Geometry check sheet. Reference: the model listing, model coordinates, mm. A direction names the side the tool comes from. Round coordinates to 2 decimals unless told otherwise and drop trailing zeros. Loops run counter-clockwise (first coordinate to the right, second up) from the corner with the lowest first, then second, coordinate; pieces in that order, holes last. Notation, with made-up numbers: (-22.5, -24.5) - (34.5, -24.5) arc R10 ccw to (34.5, -8.5) - close; hole circle Ø2 at (33.5, 18.5). An arc over 180 degrees is marked (long way). Write item = value, one per line.
```python
from build123d import *

# Parameters (mm, degrees)
SKETCH1_R           = 35
SKETCH1_R_2         = 11.65
BOSS_EXTRUDE1_DEPTH = 4
CUT_EXTRUDE1_DEPTH  = 10
SKETCH6_R           = 1
CUT_EXTRUDE4_DEPTH  = 10
BOSS_EXTRUDE3_START = 1
SKETCH7_R           = 11.65
SKETCH7_R_2         = 10.65
BOSS_EXTRUDE3_DEPTH = 1
SKETCH8_R           = 11.65
SKETCH8_R_2         = 11.15
CUT_EXTRUDE5_DEPTH  = 0.25
FILLET1_R           = 0.1
CUT_EXTRUDE6_DEPTH  = 1


with BuildPart() as part:
    # Sketch1 → Boss-Extrude1 (new body)
    with BuildSketch(Plane(origin=(0, 0, 0), x_dir=(0, -0.16775650988153862, -0.9858284604292805), z_dir=(1, 0, 0))):
        with Locations(Location((-28.542888787, 18.957113921, 0), (0, 0, 9.65740334))):
            Circle(SKETCH1_R)
        with Locations(Location((-28.542888787, 18.957113921, 0), (0, 0, 9.65740334))):
            Circle(SKETCH1_R_2, mode=Mode.SUBTRACT)
    extrude(amount=BOSS_EXTRUDE1_DEPTH)

    # Sketch2 → Cut-Extrude1 (cut)
    with BuildSketch(Plane.ZY):
        with BuildLine():
            Line((38.375552951, 38.308271509), (48.999843401, 48.932561958))
            Line((48.999843401, 48.932561958), (51.312030188, 52.930544456))
            Line((51.312030188, 52.930544456), (54.007279042, 51.111570475))
            Line((54.007279042, 51.111570475), (50.414056963, 47.518348396))
            Line((50.414056963, 47.518348396), (39.789766514, 36.894057946))
            ThreePointArc((39.789766514, 36.894057946), (39.100348464, 37.618853459), (38.375552951, 38.308271509))
        make_face()
    extrude(amount=-CUT_EXTRUDE1_DEPTH, mode=Mode.SUBTRACT)

    # Sketch6 → Cut-Extrude4 (cut)
    with BuildSketch(Plane(origin=(4, 0, 0), x_dir=(0, 0, -1), z_dir=(1, 0, 0))):
        with Locations((-24.958212841, -4.023282164)):
            Circle(SKETCH6_R)
        with Locations((2.541787159, 23.476717836)):
            Circle(SKETCH6_R)
        with Locations((-52.458212841, 23.476717836)):
            Circle(SKETCH6_R)
        with Locations((-24.958212841, 50.976717836)):
            Circle(SKETCH6_R)
    extrude(amount=-CUT_EXTRUDE4_DEPTH, mode=Mode.SUBTRACT)

    # Sketch7 → Boss-Extrude3 (add)
    with BuildSketch(Plane.ZY.offset(-4).offset(BOSS_EXTRUDE3_START)):
        with Locations((24.958212841, 23.476717836)):
            Circle(SKETCH7_R)
        with Locations((24.958212841, 23.476717836)):
            Circle(SKETCH7_R_2, mode=Mode.SUBTRACT)
    extrude(amount=-BOSS_EXTRUDE3_DEPTH)

    # Sketch8 → Cut-Extrude5 (cut)
    with BuildSketch(Plane.ZY.offset(-3)):
        with Locations((24.958212841, 23.476717836)):
            Circle(SKETCH8_R)
        with Locations((24.958212841, 23.476717836)):
            Circle(SKETCH8_R_2, mode=Mode.SUBTRACT)
    extrude(amount=-CUT_EXTRUDE5_DEPTH, mode=Mode.SUBTRACT)

    # Fillet1
    fillet1_edges = [part.edges().sort_by_distance(p)[0] for p in [
        (3.25, 23.476717836, 13.808212841),
    ]]
    fillet(fillet1_edges, radius=FILLET1_R)

    # Sketch9 → Cut-Extrude6 (cut)
    with BuildSketch(Plane.ZY):
        Polygon((36.254232608, 38.308271509), (48.989739813, 51.043778714), (52.525273719, 47.508244808), (39.789766514, 34.772737603), (39.082659732, 34.065630822), (35.547125827, 37.601164728), align=None)
        Polygon((48.989739813, 48.922458371), (50.403953376, 47.508244808), (40.402946038, 37.507237471), (38.988732476, 38.921451033), align=None, mode=Mode.SUBTRACT)
    extrude(amount=-CUT_EXTRUDE6_DEPTH, mode=Mode.SUBTRACT)


solid = part.part
```
(1) Section check C-C (z = 9.5). Enter the section's corners in (x, y), then the cut area to 3 significant figures.
Answers follow:
outline = (0, -7.92) - (4, -7.92) - (4, 54.88) - (0, 54.88) - close
area = 251 mm²
(2) Scan lines: L1, parallel to Y at x = 3.05, z = 26; L2, parallel to Y at x = 2.9, z = 16; L3, parallel to X at y = 48, z = 46. Record each from-to range of solid material in increasing order. Write a range as [from, to].
Answers follow:
L1 = [-11.51, 11.87], [12.38, 12.88], [34.08, 34.58], [35.08, 58.46]
L2 = [-10.36, 16.03], [30.92, 57.31]
L3 = [1, 4]
(3) Mould release check, pull along Z, two halves, no side actions. Record for faces 1 (the flat face through (4, 16, 17)), 2 (the flat face through (2.479, 42.275, 45.171)): pulls with the +Z half, pulls with the -Z half, needs draft (parallel to the pull), parting line crosses it, or undercut.
Answers follow:
face_1 = needs draft
face_2 = undercut
(4) Set-up check for faces 3 (the flat face through (2.48, 43.54, 43.61)), 4 (the flat face through (0, 24, 10)), 5 (the flat face through (1, 40, 44)): record each of +Z, -Z, +X, -X, +Y, -Y from which the full face is reachable in a straight line by a thin tool's end or side.
Answers follow:
face_3 = +X, -X
face_4 = +Z, -Z, -X, +Y, -Y
face_5 = -X
(5) Gauge pin test, flat ends, axial feed: pin 1 (2 mm diameter, centred on x = 3.5, z = 31.5, fed in from -Y); pin 2 (1.6 mm diameter, centred on y = -4.02, z = 24.96, fed in from -X); pin 3 (1 mm diameter, centred on x = 3, z = 34.5, fed in from -Y). Record the tip position at first contact, or that the pin passes through.
Answers follow:
pin_1 = -11.08
pin_2 = through
pin_3 = -10.34
(6) Section check A-A (y = 42). Enter the section's corners in (x, z), then the cut area to 3 significant figures.
Answers follow:
outline = (0, -4.74) - (4, -4.74) - (4, 42.07) - (1, 42.07) - (1, 39.95) - (0, 39.95) - close; (0, 47.02) - (1, 47.02) - (1, 44.9) - (4, 44.9) - (4, 54.65) - (0, 54.65) - close
area = 222 mm²
(7) Section check B-B (x = 1.75). Enter the section's corners in (y, z).
Answers follow:
outline = (36.89, 39.79) - (47.51, 50.4) arc R35 ccw (long way) to (48.92, 48.99) - (38.31, 38.38) arc R20 ccw to start; hole circle Ø2 at (-4.02, 24.96); hole circle Ø23.3 at (23.48, 24.96); hole circle Ø2 at (23.48, -2.54); hole circle Ø2 at (23.48, 52.46); hole circle Ø2 at (50.98, 24.96)
